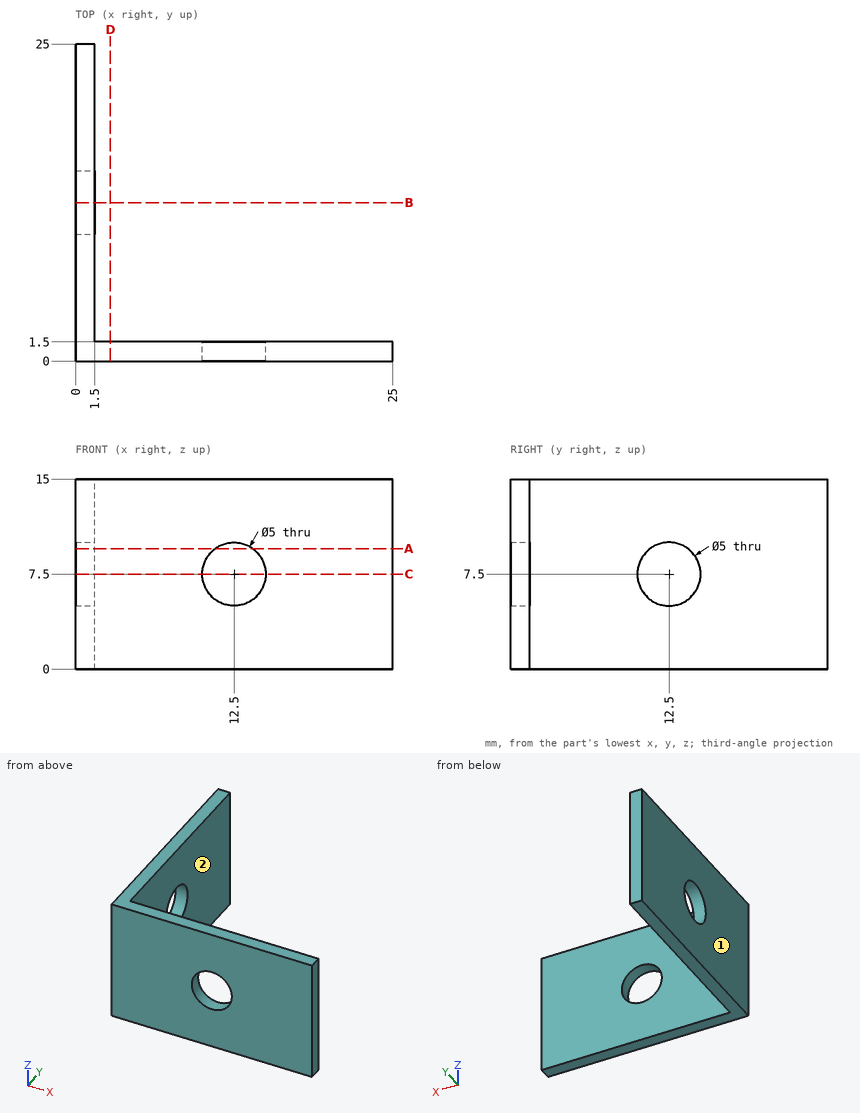
Input: dimensioned drawing with shaded views. Units: mm. Origin: part minimum x, y, z. A direction names the side the tool comes from. Round coordinates to 2 decimals unless told otherwise and drop trailing zeros. Order: outer loops, then holes, each group sorted by start corner. A loop starts at its lowest first (then second) coordinate and runs counter-clockwise, first axis right, second up. Notation, with made-up numbers: (0, 48.5) - (38, 48.5) arc R27 ccw to (38, 74.5) - close; hole circle Ø4 at (48, 22.25). An arc over 180 degrees is marked (long way). Use CSV: the item, a comma, the result in double quotes. Start each with the question number.
Q1. Material intervals for line 1 along Z through (x, y) = (0.9, 12.5); line 2 along Y through (x, z) = (0.75, 7.5), sorted ascending. Write a range as from..to.
Q2. Section query B-B (y = 12.5). Return loops of the section in (x, z).
Q3. Access query for the marked faces 1 and 2. Directions: +Z, -Z, +X, -X, +Y, -Y. A direction counts if a zero-diameter tool reaches every point of the face in a straight line with its end or side. Return the directions, or none.
Q4. Section query C-C (z = 7.5). Return loops of the section in (x, y).
Q5. First-contact query: pin 1 (3 mm diameter, centred on y = 13.5, z = 8.5, fed in from +X); pin 2 (5 mm diameter, centred on x = 4.5, y = 16.5, fed in from -Z); pin 3 (4 mm diameter, centred on x = 18.5, z = 6, fed in from +Y). Flat tips, straight axial feed; report the tip coordinate or a pass-through.
Q6. Section query D-D (x = 2.75). Return loops of the section in (y, z).
Q7. Section query A-A (z = 9.5). Return loops of the section in (x, y), and give its area (4 significant figures).
Result set:
1,line 1,"z = 0..5, 10..15"
1,line 2,"y = 0..10, 15..25"
2,outline,"(0, 0) - (1.5, 0) - (1.5, 5) - (0, 5) - close; (0, 10) - (1.5, 10) - (1.5, 15) - (0, 15) - close"
3,face 1,"+Z, -Z, -X, +Y, -Y"
3,face 2,"+Z, -Z, +X, +Y"
4,outline,"(0, 0) - (10, 0) - (10, 1.5) - (1.5, 1.5) - (1.5, 10) - (0, 10) - close; (0, 15) - (1.5, 15) - (1.5, 25) - (0, 25) - close; (15, 0) - (25, 0) - (25, 1.5) - (15, 1.5) - close"
5,pin 1,"stops at x = 1.5"
5,pin 2,"passes through"
5,pin 3,"stops at y = 1.5"
6,outline,"(0, 0) - (1.5, 0) - (1.5, 15) - (0, 15) - close"
7,outline,"(0, 0) - (11, 0) - (11, 1.5) - (1.5, 1.5) - (1.5, 11) - (0, 11) - close; (0, 14) - (1.5, 14) - (1.5, 25) - (0, 25) - close; (14, 0) - (25, 0) - (25, 1.5) - (14, 1.5) - close"
7,area,"63.75 mm2"
